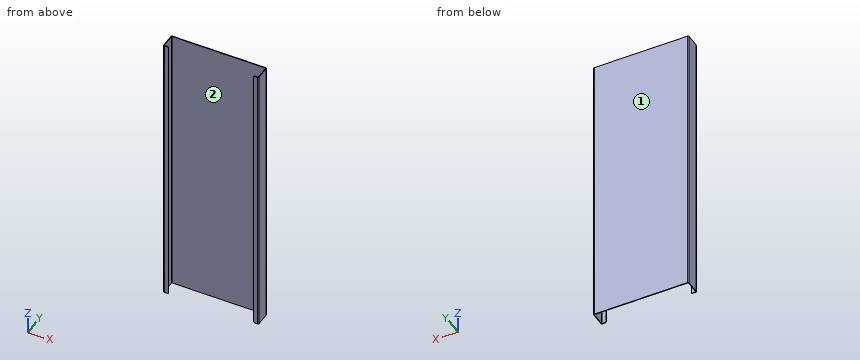
from build123d import *

# Parameters (mm, degrees)
F1_DEPTH = 373.5
F2_R     = 2


with BuildPart() as f1:
    # F0 (on Top) → F1 (new body, symmetric)
    with BuildSketch(Plane.XY):
        with BuildLine():
            Line((122.5, 0), (0, 0))
            Line((0, 0), (-122.5, 0))
            ThreePointArc((-122.5, 0), (-124.267767, -0.732233), (-125, -2.5))
            Line((-125, -2.5), (-125, -37.5))
            ThreePointArc((-125, -37.5), (-124.267767, -39.267767), (-122.5, -40))
            Line((-122.5, -40), (-112, -40))
            Line((-112, -40), (-112, -38.5))
            Line((-112, -38.5), (-122.5, -38.5))
            ThreePointArc((-122.5, -38.5), (-123.207107, -38.207107), (-123.5, -37.5))
            Line((-123.5, -37.5), (-123.5, -2.5))
            ThreePointArc((-123.5, -2.5), (-123.207107, -1.792893), (-122.5, -1.5))
            Line((-122.5, -1.5), (0, -1.5))
            Line((0, -1.5), (122.5, -1.5))
            ThreePointArc((122.5, -1.5), (123.207107, -1.792893), (123.5, -2.5))
            Line((123.5, -2.5), (123.5, -37.5))
            ThreePointArc((123.5, -37.5), (123.207107, -38.207107), (122.5, -38.5))
            Line((122.5, -38.5), (112, -38.5))
            Line((112, -38.5), (112, -40))
            Line((112, -40), (122.5, -40))
            ThreePointArc((122.5, -40), (124.267767, -39.267767), (125, -37.5))
            Line((125, -37.5), (125, -2.5))
            ThreePointArc((125, -2.5), (124.267767, -0.732233), (122.5, 0))
        make_face()
    extrude(amount=F1_DEPTH, both=True)

    # F2
    f2_edges = [f1.edges().sort_by_distance(p)[0] for p in [
        (-112, -39.25, -373.5),
        (112, -39.25, -373.5),
        (112, -39.25, 373.5),
        (-112, -39.25, 373.5),
    ]]
    fillet(f2_edges, radius=F2_R)


solid = f1.part
Geometry: final body of the model. Coordinates: model frame, mm. Face numbers are marked on the shaded views. Give positions to 0.01 mm unless a question says otherwise; leave off trailing zeros. Write each loop counter-clockwise with the first axis right and the second up, starting at its lowest first coordinate (ties: lowest second). Pieces come first, ordered by that corner, then holes. Notation, with made-up numbers: M -31,-40 L 1,-40 A19 ccw 1,-18 Z; hole C 85,88 d7. An arc over 180 degrees is marked long. Answer in a Markdown table with one row per item. Add a question column.
(1) Section C-C on x = 36. Return loops of the section in (y, z).
(2) First-contact query: pin 1 (5 mm diameter, centred on x = 93, y = -5.5, fed in from -Z); pin 2 (1.6 mm diameter, centred on y = -39, z = 27.5, fed in from -X); pin 3 (5 mm diameter, centred on x = 29, z = -142.5, fed in from -Y). Flat tips, straight axial feed; report the tip coordinate or a pass-through.
(3) Section B-B on z = 197. Return loops of the section in (x, y).
(4) Mould query, pull axis X, two halves, no side actions, for the marked faces 1 and 2. Classes: +X half, -X half, draft (parallel to the pull), parting line (faces both ways), or undercut.
(5) Ray query, line 1 (X direction, y = -36.5, z = -88.5); line 2 (Y direction, x = -54.5, z = 90); line 3 (X direction, y = -2, z = 52.5). Return the intervals inside material, ascending.
(6) Section A-A on y = -23. Return loops of the section in (x, z).
Result set:
| question | item | result |
|---|---|---|
| 1 | outline | M -1.5,-373.5 L 0,-373.5 L 0,373.5 L -1.5,373.5 Z |
| 2 | pin 1 | passes through |
| 2 | pin 2 | stops at x = -124.9 |
| 2 | pin 3 | stops at y = -1.5 |
| 3 | outline | M -125,-37.5 A2.5 ccw -122.5,-40 L -112,-40 L -112,-38.5 L -122.5,-38.5 A1 cw -123.5,-37.5 L -123.5,-2.5 A1 cw -122.5,-1.5 L 122.5,-1.5 A1 cw 123.5,-2.5 L 123.5,-37.5 A1 cw 122.5,-38.5 L 112,-38.5 L 112,-40 L 122.5,-40 A2.5 ccw 125,-37.5 L 125,-2.5 A2.5 ccw 122.5,0 L -122.5,0 A2.5 ccw -125,-2.5 Z |
| 4 | face 1 | draft |
| 4 | face 2 | undercut |
| 5 | line 1 | x = -125 to -123.5, 123.5 to 125 |
| 5 | line 2 | y = -1.5 to 0 |
| 5 | line 3 | x = -124.95 to -123.37, 123.37 to 124.95 |
| 6 | outline | M -125,-373.5 L -123.5,-373.5 L -123.5,373.5 L -125,373.5 Z; M 123.5,-373.5 L 125,-373.5 L 125,373.5 L 123.5,373.5 Z |
